from build123d import *

# Parameters (mm, degrees)
SKIZZE9_W                       = 220
SKIZZE9_H                       = 575
BASIS_BLECH2_DEPTH              = 2
KANTE_LASCHE3_STRIP_W           = 8.2
KANTE_LASCHE3_STRIP_H           = 2
KANTE_LASCHE3_STRIP_CUT_DEPTH   = 575
KANTE_LASCHE3_DEPTH             = 575
KANTE_LASCHE3_FLAT_DEPTH        = 2
KANTE_LASCHE4_STRIP_CUT_DEPTH   = 217.9
KANTE_LASCHE4_STRIP_CUT_2_DEPTH = 217.9
KANTE_LASCHE4_DEPTH             = 217.9
KANTE_LASCHE4_BEND_DEPTH        = 217.9
SKIZZE43_W                      = 10
SKIZZE43_H                      = 42
SCHNITT_LINEAR_AUSTRAGEN4_DEPTH = 326.18077275
KANTE_LASCHE5_DEPTH             = 574.994641016


# Sheet-metal steps are written as plain solids
with BuildPart() as part:
    # Skizze9 → Basis-Blech2 (new body)
    with BuildSketch(Plane(origin=(0, 0, 0), x_dir=(1, 0, 0), z_dir=(0, 1, 0))):
        Rectangle(SKIZZE9_W, SKIZZE9_H)
    extrude(amount=-BASIS_BLECH2_DEPTH)

    # Kante-Lasche3 strip (across the edge) → Kante-Lasche3 strip cut (cut)
    with BuildSketch(Plane(origin=(110, -2, -287.5), x_dir=(-1, 0, 0), z_dir=(0, 0, 1))):
        with Locations((-2, -1)):
            Rectangle(KANTE_LASCHE3_STRIP_W, KANTE_LASCHE3_STRIP_H)
    extrude(amount=KANTE_LASCHE3_STRIP_CUT_DEPTH, mode=Mode.SUBTRACT)

    # Kante-Lasche3 bend section (across the edge) → Kante-Lasche3 (add)
    with BuildSketch(Plane(origin=(110, -2, -287.5), x_dir=(-1, 0, 0), z_dir=(0, 0, 1))):
        with BuildLine():
            Line((0, 0.1), (2, 0.1))
            ThreePointArc((2, 0.1), (2.029289322, 0.029289322), (2.1, 0))
            Line((2.1, 0), (2.1, -2))
            ThreePointArc((2.1, -2), (0.61507576, -1.38492424), (0, 0.1))
        make_face()
    extrude(amount=KANTE_LASCHE3_DEPTH)

    # Kante-Lasche3 profile (on flange) → Kante-Lasche3 flat (add)
    with BuildSketch(Plane(origin=(110, -2, 0), x_dir=(0, 0, 1), z_dir=(1, 0, 0))):
        with BuildLine():
            Line((287.5, 0.1), (287.5, 7))
            Line((287.5, 7), (245.5, 7))
            ThreePointArc((245.5, 7), (241.964466094, 8.464466094), (240.5, 12))
            Line((240.5, 12), (240.5, 18))
            Line((240.5, 18), (127.7, 18))
            Line((127.7, 18), (127.7, 10))
            ThreePointArc((127.7, 10), (125, 7.3), (122.3, 10))
            Line((122.3, 10), (122.3, 18))
            Line((122.3, 18), (2.7, 18))
            Line((2.7, 18), (2.7, 10))
            ThreePointArc((2.7, 10), (0, 7.3), (-2.7, 10))
            Line((-2.7, 10), (-2.7, 18))
            Line((-2.7, 18), (-122.3, 18))
            Line((-122.3, 18), (-122.3, 10))
            ThreePointArc((-122.3, 10), (-125, 7.3), (-127.7, 10))
            Line((-127.7, 10), (-127.7, 18))
            Line((-127.7, 18), (-240.5, 18))
            Line((-240.5, 18), (-240.5, 12))
            ThreePointArc((-240.5, 12), (-241.964466094, 8.464466094), (-245.5, 7))
            Line((-245.5, 7), (-287.5, 7))
            Line((-287.5, 7), (-287.5, 0.1))
            Line((-287.5, 0.1), (287.5, 0.1))
        make_face()
    extrude(amount=-KANTE_LASCHE3_FLAT_DEPTH)

    # Kante-Lasche4 strip (across the edge) → Kante-Lasche4 strip cut (cut)
    with BuildSketch(Plane(origin=(-110, -2, -287.5), x_dir=(0, -0.8660254037844416, 0.49999999999999495), z_dir=(1, 0, 0))):
        Polygon((-5.740711062, 5.94320323), (-1.730711062, -1.002320508), (0.001339746, -0.002320508), (-4.008660254, 6.94320323), align=None)
    extrude(amount=KANTE_LASCHE4_STRIP_CUT_DEPTH, mode=Mode.SUBTRACT)

    # Kante-Lasche4 strip 2 (across the edge) → Kante-Lasche4 strip cut 2 (cut)
    with BuildSketch(Plane(origin=(107.9, -2, 287.5), x_dir=(0, -0.8660254037844416, -0.49999999999999495), z_dir=(-1, 0, 0))):
        Polygon((-5.740711062, 5.94320323), (-1.730711062, -1.002320508), (0.001339746, -0.002320508), (-4.008660254, 6.94320323), align=None)
    extrude(amount=KANTE_LASCHE4_STRIP_CUT_2_DEPTH, mode=Mode.SUBTRACT)

    # Kante-Lasche4 section (across the edge) → Kante-Lasche4 (add)
    with BuildSketch(Plane(origin=(-110, -2, -287.5), x_dir=(0, -0.8660254037844416, 0.49999999999999495), z_dir=(1, 0, 0))):
        with BuildLine():
            Line((-2, 0.002679492), (-2, 19.464101615))
            Line((-2, 19.464101615), (0, 19.464101615))
            Line((0, 19.464101615), (0, 0.002679492))
            ThreePointArc((0, 0.002679492), (0.000340742, 9.1301e-05), (0.001339746, -0.002320508))
            Line((0.001339746, -0.002320508), (-1.730711062, -1.002320508))
            ThreePointArc((-1.730711062, -1.002320508), (-1.931510911, -0.517546789), (-2, 0.002679492))
        make_face()
    extrude(amount=KANTE_LASCHE4_DEPTH)

    # Kante-Lasche4 section 2 (across the edge) → Kante-Lasche4 bend (add)
    with BuildSketch(Plane(origin=(107.9, -2, 287.5), x_dir=(0, -0.8660254037844416, -0.49999999999999495), z_dir=(-1, 0, 0))):
        with BuildLine():
            Line((-2, 0.002679492), (-2, 19.464101615))
            Line((-2, 19.464101615), (0, 19.464101615))
            Line((0, 19.464101615), (0, 0.002679492))
            ThreePointArc((0, 0.002679492), (0.000340742, 9.1301e-05), (0.001339746, -0.002320508))
            Line((0.001339746, -0.002320508), (-1.730711062, -1.002320508))
            ThreePointArc((-1.730711062, -1.002320508), (-1.931510911, -0.517546789), (-2, 0.002679492))
        make_face()
    extrude(amount=KANTE_LASCHE4_BEND_DEPTH)

    # Skizze43 → Schnitt-Linear austragen4 (cut, through all)
    with BuildSketch(Plane(origin=(0, 0, 0), x_dir=(1, 0, 0), z_dir=(0, 1, 0))):
        with Locations((105, 287.497320508)):
            Rectangle(SKIZZE43_W, SKIZZE43_H)
        with Locations((105, -287.497320508)):
            Rectangle(SKIZZE43_W, SKIZZE43_H)
    extrude(amount=-SCHNITT_LINEAR_AUSTRAGEN4_DEPTH, mode=Mode.SUBTRACT)

    # Kante-Lasche5 section (across the edge) → Kante-Lasche5 (add)
    with BuildSketch(Plane(origin=(-110.083909963, -2, 287.497320508), x_dir=(0.9848077530122075, -0.17364817766693427, 0), z_dir=(0, 0, -1))):
        with BuildLine():
            Line((-2, 0.083909963), (-2, 7))
            Line((-2, 7), (0, 7))
            Line((0, 7), (0, 0.083909963))
            ThreePointArc((0, 0.083909963), (0.023395556, 0.019631202), (0.082635182, -0.014570812))
            Line((0.082635182, -0.014570812), (-0.264661173, -1.984186318))
            ThreePointArc((-0.264661173, -1.984186318), (-1.508693331, -1.265944017), (-2, 0.083909963))
        make_face()
    extrude(amount=KANTE_LASCHE5_DEPTH)


solid = part.part
The model under review builds one solid part; all positions refer to its coordinate system, in mm. A direction names the side the tool comes from. Coordinates: 2 decimals unless noted, no trailing zeros. Write each loop counter-clockwise with the first axis right and the second up, starting at its lowest first coordinate (ties: lowest second). Pieces come first, ordered by that corner, then holes. Notation, with made-up numbers: M 68.5,21.25 L 105.5,21.25 A24 cw 105.5,60.25 Z; hole C 8.25,-29.5 d6. An arc over 180 degrees is marked long. Put each result on its own line as item: value.
1) Draft analysis for pull direction Z (two halves, no side actions). For faces 1 (the flat face through (-6.47, -5.067, -296.811)), 2 (the flat face through (-110, -6, 296)), 3 (the flat face through (-3, -2, -4)), state which applies: released by +Z, released by -Z, zero draft, split by the parting line, or undercut.
Computed:
face 1: released by -Z
face 2: zero draft
face 3: undercut
2) Clearance check with flat-ended pins moving along their axes: pin 1 Ø12 at (x, y) = (39.5, -17) entering from -Z; pin 2 Ø6 at (y, z) = (-4.5, -295.5) entering from -X; pin 3 Ø1.6 at (x, y) = (109, -16.5) entering from -Z. State where each tip first meets the part, or that it passes through.
Computed:
pin 1: stops at z = -304.78
pin 2: stops at x = -110
pin 3: stops at z = -240.5
3) For faces 4 (the flat face through (108, -11, -4)), 5 (the flat face through (100, -1, 286)), 6 (the flat face through (100, -1, -286)), list the 3-axis set-ups (+Z, -Z, +X, -X, +Y, -Y) from which the entire face can be reached by the end or side of a thin tool; tool diameter is ignored.
Computed:
face 4: +Z, -Z, -Y
face 5: +Z, +X, +Y, -Y
face 6: -Z, +X, +Y, -Y
4) Add section A-A on z = 10.5. Give the boundary of the cut face in (x, y), then the cut area to 3 significant figures.
Computed:
outline: M -113.27,-8.55 L -111.3,-8.89 L -110.1,-2.08 A0.1 cw -110,-2 L 107.9,-2 A0.1 cw 108,-2.1 L 108,-20 L 110,-20 L 110,-2.1 A2.1 ccw 107.9,0 L -110,0 A2.1 ccw -112.07,-1.74 Z
area: 492 mm2
5) Wall thickness on probe 1 along X at (y, z) = (-2.25, -51.5); probe 2 along X at (y, z) = (-1.75, 142.5); probe 3 along X at (y, z) = (-18, -89.5): over which ranges is each line inside the solid? List them lowest first. Write a range as [from, to].
Computed:
probe 1: x = [-112.16, -110.13], [108, 110]
probe 2: x = [-112.07, 109.97]
probe 3: x = [108, 110]
